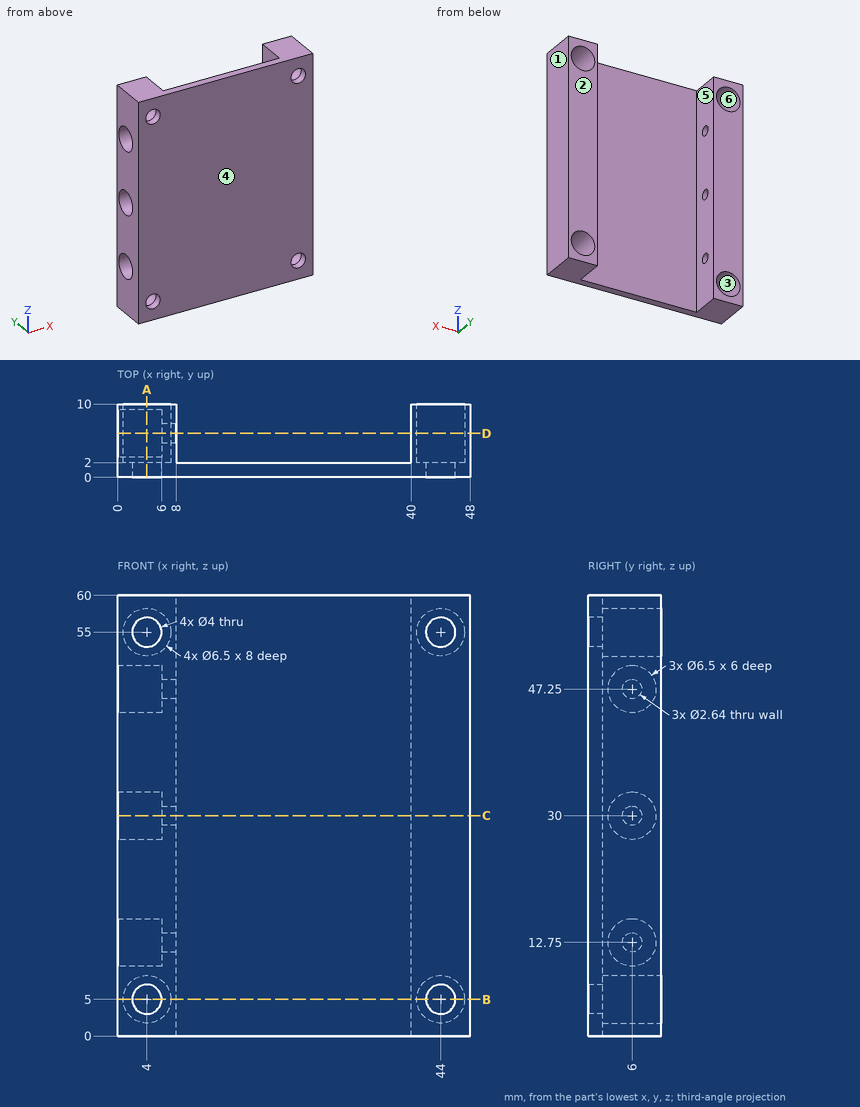
Input: dimensioned drawing with shaded views. Units: mm. Origin: part minimum x, y, z. A direction names the side the tool comes from. Give positions to 0.01 mm unless a question says otherwise; leave off trailing zeros. Write each loop counter-clockwise with the first axis right and the second up, starting at its lowest first coordinate (ties: lowest second). Pieces come first, ordered by that corner, then holes.
Q1. Set-up query: the marked faces 4, 5 and 6. Return all of +Z, -Z, +X, -X, +Y, -Y with unobstructed straight access to the full face (end or side cutting, diameter ignored); none if empty.
Q2. Material intervals for probe 1 along X at (y, z) = (6.25, 55); probe 2 along Z at (x, y) = (4, 0.45); probe 3 along X at (y, z) = (5.5, 21), sorted ascending.
Q3. Pull-direction query (X, two-part tool) for the marked faces 1, 2 and 3; classes: pulls with the +X half, pulls with the -X half, needs draft (parallel to the pull), parting line crosses it, or undercut.
Q4. Section C-C, the plane z = 30. Output: boundary loops of the cut face in (x, y).
Q5. Section D-D, the plane y = 6. State how many separate pieces and enclosed holes the cut face has, plus the area to 3 significant figures.
Q6. Section B-B, the plane z = 5. Output: boundary loops of the cut face in (x, y), plus the area to 3 significant figures.
Q7. First-contact query: P1, Ø2, axis at x = 43.5, z = 4, coming from the +Y side; P2, Ø2, axis at y = 6.5, z = 13.5, coming from the -X side. Flat tips, straight axial feed; report the tip coordinate or a pass-through.
Q8. Section A-A, the plane x = 4. Output: boundary loops of the cut face in (y, z), plus the area to 3 significant figures.
Filled in:
1. face 4: +Z, -Z, +X, -X, -Y
1. face 5: +Z, -Z, +Y
1. face 6: +Y
2. probe 1: x = 0 to 0.75, 7.25 to 8, 40 to 40.75, 47.25 to 48
2. probe 2: z = 0 to 3, 7 to 53, 57 to 60
2. probe 3: x = 0 to 8, 40 to 48
3. face 1: pulls with the +X half
3. face 2: needs draft
3. face 3: undercut
4. outline: (0, 0) - (48, 0) - (48, 10) - (40, 10) - (40, 2) - (8, 2) - (8, 4.68) - (6, 4.68) - (6, 2.75) - (0, 2.75) - close; (0, 9.25) - (6, 9.25) - (6, 7.32) - (8, 7.32) - (8, 10) - (0, 10) - close
5. separate pieces: 5
5. enclosed holes: 4
5. area: 694 mm2
6. outline: (0, 0) - (2, 0) - (2, 2) - (0.75, 2) - (0.75, 10) - (0, 10) - close; (6, 0) - (42, 0) - (42, 2) - (40.75, 2) - (40.75, 10) - (40, 10) - (40, 2) - (8, 2) - (8, 10) - (7.25, 10) - (7.25, 2) - (6, 2) - close; (46, 0) - (48, 0) - (48, 10) - (47.25, 10) - (47.25, 2) - (46, 2) - close
6. area: 104 mm2
7. P1: stops at y = 2
7. P2: stops at x = 6
8. outline: (0, 0) - (10, 0) - (10, 1.75) - (2, 1.75) - (2, 3) - (0, 3) - close; (0, 7) - (2, 7) - (2, 8.25) - (10, 8.25) - (10, 51.75) - (2, 51.75) - (2, 53) - (0, 53) - close; (0, 57) - (2, 57) - (2, 58.25) - (10, 58.25) - (10, 60) - (0, 60) - close; hole circle Ø6.5 at (6, 12.75); hole circle Ø6.5 at (6, 30); hole circle Ø6.5 at (6, 47.25)
8. area: 380 mm2
